```python
from build123d import *

# Parameters (mm, degrees)
SKETCH_1_R                   = 8
EXTRUDE_1_DEPTH              = 25.5
SKETCH_2_W                   = 1
SKETCH_2_H                   = 10
CUT_EXTRUDE_2_DEPTH          = 9.25
HOLE_WIZARD_M8_1_D           = 6.8
HOLE_WIZARD_M8_1_DEPTH       = 19.75
HOLE_WIZARD_M8_1_CBORE_D     = 8
HOLE_WIZARD_M8_1_CBORE_DEPTH = 16
HOLE_WIZARD_M8_1_TIP         = 2.042926105
SKETCH_4_R                   = 4
EXTRUDE_3_DEPTH              = 12
CHAMFER_1_SIZE               = 0.5
SKETCH_5_W                   = 1.5
SKETCH_5_H                   = 0.930014358


with BuildPart() as part:
    # 草图1 → 拉伸1 (new body)
    with BuildSketch(Plane.XY):
        Circle(SKETCH_1_R)
    extrude(amount=EXTRUDE_1_DEPTH)

    # 草图2 → 拉伸2 (cut, symmetric)
    with BuildSketch(Plane(origin=(0, 0, 0), x_dir=(1, 0, 0), z_dir=(0, 1, 0))):
        with Locations((-7.5, -10)):
            Rectangle(SKETCH_2_W, SKETCH_2_H)
        with Locations((7.5, -10)):
            Rectangle(SKETCH_2_W, SKETCH_2_H)
    extrude(amount=CUT_EXTRUDE_2_DEPTH, both=True, mode=Mode.SUBTRACT)

    # M8 螺纹孔1
    with Locations(Plane(origin=(0, 0, 0), x_dir=(-1, 0, 0), z_dir=(0, 0, -1))):
        with Locations((0, 0)):
            CounterBoreHole(HOLE_WIZARD_M8_1_D / 2, HOLE_WIZARD_M8_1_CBORE_D / 2, HOLE_WIZARD_M8_1_CBORE_DEPTH, depth=HOLE_WIZARD_M8_1_DEPTH)
            with Locations((0, 0, -(HOLE_WIZARD_M8_1_DEPTH + HOLE_WIZARD_M8_1_TIP / 2))):  # 118° drill point
                Cone(0, HOLE_WIZARD_M8_1_D / 2, HOLE_WIZARD_M8_1_TIP, mode=Mode.SUBTRACT)

    # 草图4 → 拉伸3 (add)
    with BuildSketch(Plane.XY.offset(25.5)):
        with Locations(Location((0, 0, 0), (0, 0, 180))):
            Circle(SKETCH_4_R)
    extrude(amount=EXTRUDE_3_DEPTH)

    # 倒角1
    chamfer_1_edges = [part.edges().sort_by_distance(p)[0] for p in [
        (4, 0, 37.5),
    ]]
    chamfer(chamfer_1_edges, length=CHAMFER_1_SIZE)

    # 草图5 → 切除-旋转1 (revolve, cut)
    with BuildSketch(Plane(origin=(0, 0, 0), x_dir=(0, 0, -1), z_dir=(1, 0, 0)), mode=Mode.PRIVATE) as cut_revolve_1_sk:
        with Locations((-26.25, 3.965007179)):
            Rectangle(SKETCH_5_W, SKETCH_5_H)
    revolve(cut_revolve_1_sk.sketch.rotate(Axis((0, 0, 25.5), (0, 0, -1)), 270), axis=Axis((0, 0, 25.5), (0, 0, -1)), mode=Mode.SUBTRACT)


solid = part.part
```
Here's how the part is built. I have some questions about the finished solid (model axes, mm). A direction names the side the tool comes from. Give positions to 0.01 mm unless a question says otherwise; leave off trailing zeros. Order: outer loops, then holes, each group sorted by start corner. A loop starts at its lowest first (then second) coordinate and runs counter-clockwise, first axis right, second up. Notation, with made-up numbers: (55.25, -7.75) - (86.25, -7.75) arc R22 cw to (86.25, 16.25) - close; hole circle Ø2 at (79.5, 11). An arc over 180 degrees is marked (long way). Answer as a JSON object with one key per item and string values. Group by question number.
Item 1: If we section it at A-A on z = 12: Please give me the cut outline in (x, y), and give its area (3 significant figures).
Item 2: If we section it at D-D on y = 6: Please give me the cut outline in (x, z).
Item 3: Please list where these lines run through material, in increasing order: probe 1 along X at (y, z) = (0, 18.1); probe 2 along Y at (x, z) = (0, 4); probe 3 along Z at (x, y) = (2, -6.75).
Item 4: Which directions (+Z, -Z, +X, -X, +Y, -Y) give clear straight access to the entire face, cutting with the end or side of a thin tool? Please do faces 1 (the cylindrical face through (0.759, -3.417, 26.24)), 2 (the flat face through (-7, 0, 10)), 3 (the flat face through (7.4, 0.1, 5)).
Item 5: For P1, Ø8, axis at x = -5, z = 16, coming from the +Y side; P2, Ø1, axis at y = 1.5, z = 29, coming from the -X side; P3, Ø4, axis at y = 0.5, z = 12, coming from the -X side; P4, Ø9, axis at x = 0.5, y = 1, coming from the -Z side, each with a flat end and sliding along its axis, tell me the tip position at first contact or that it passes through.
Item 6: If we section it at B-B on z = 32: Please give me the cut outline in (x, y).
Item 7: If we mould it in two halves opening along Z, with no side actions, what happens to faces 4 (the cylindrical face through (-0.74, -3.32, 17.9)), 5 (the flat face through (7.4, 0.1, 15)), 6 (the flat face through (0, 0, 37.5))? For each: pulls with the +Z half, pulls with the -Z half, needs draft (parallel to the pull), parting line crosses it, or undercut.
Item 8: If we section it at C-C on x = 5.5: Please give me the cut outline in (y, z).
Result set:
{
 "1": {"outline": "(-7, -3.87) arc R8 ccw to (7, -3.87) - (7, 3.87) arc R8 ccw to (-7, 3.87) - close; hole circle Ø8 at (0, 0)", "area": "140 mm²"},
 "2": {"outline": "(-5.29, 0) - (5.29, 0) - (5.29, 25.5) - (-5.29, 25.5) - close"},
 "3": {"probe 1": "-8 to -3.4, 3.4 to 8", "probe 2": "-8 to -4, 4 to 8", "probe 3": "0 to 25.5"},
 "4": {"face 1": "none", "face 2": "-X, +Y, -Y", "face 3": "+X, +Y, -Y"},
 "5": {"P1": "y = 7.94", "P2": "x = -3.87", "P3": "x = -7", "P4": "z = 0"},
 "6": {"outline": "circle Ø8 at (0, 0)"},
 "7": {"face 4": "needs draft", "face 5": "undercut", "face 6": "pulls with the +Z half"},
 "8": {"outline": "(-5.81, 0) - (5.81, 0) - (5.81, 25.5) - (-5.81, 25.5) - close"}
}
